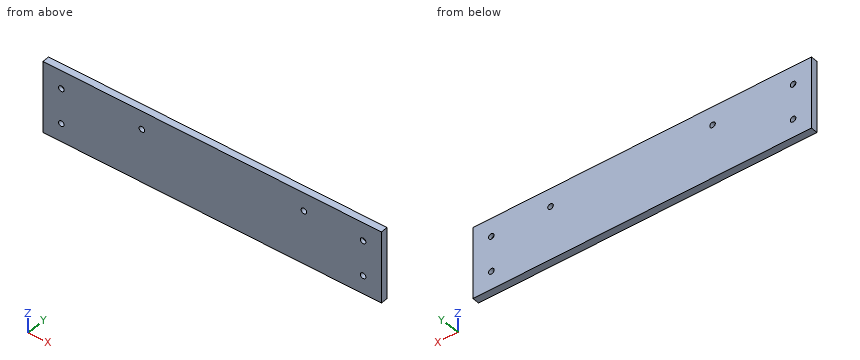
```python
from build123d import *

# Parameters (mm, degrees)
SKETCH1_W               = 305
SKETCH1_H               = 65
BOSS_EXTRUDE1_DEPTH     = 3.175
SKETCH4_R               = 2.5
CUT_EXTRUDE2_DEPTH      = 159.40243251
CUT_EXTRUDE3_DEPTH      = 157.053908955
CUT_EXTRUDE3_DEPTH_BACK = 157.053908955
SKETCH5_R               = 2.5


with BuildPart() as part:
    # Sketch1 → Boss-Extrude1 (new, symmetric)
    with BuildSketch(Plane(origin=(0, 0, 0), x_dir=(1, 0, 0), z_dir=(0, 1, 0))):
        Rectangle(SKETCH1_W, SKETCH1_H)
    extrude(amount=BOSS_EXTRUDE1_DEPTH, both=True)

    # Sketch4 → Cut-Extrude2 (cut, symmetric)
    with BuildSketch(Plane(origin=(-2.5, 0, 0), x_dir=(-1, 0, 0), z_dir=(0, -1, 0))):
        with Locations(Location((133.48, -15.98, 0), (0, 0, 90))):
            Circle(SKETCH4_R)
        with Locations(Location((133.48, 15.98, 0), (0, 0, 270))):
            Circle(SKETCH4_R)
    cut_extrude2 = extrude(amount=CUT_EXTRUDE2_DEPTH, both=True, mode=Mode.SUBTRACT)

    # Mirror2: Cut-Extrude2 across plane
    add(cut_extrude2.mirror(Plane(origin=(0, 0, 0), x_dir=(0, 0, 1), z_dir=(1, 0, 0))), mode=Mode.SUBTRACT)

    # Sketch5 → Cut-Extrude3 (cut, two sides: drawn at the far end of the back side and taken through both)
    with BuildSketch(Plane(origin=(0, 3.175, 0), x_dir=(1, 0, 0), z_dir=(0, 1, 0)).offset(-CUT_EXTRUDE3_DEPTH_BACK)):
        with Locations(Location((82.64, -15.98, 0), (0, 0, 270))):
            Circle(SKETCH5_R)
        with Locations(Location((-63.41, -15.98, 0), (0, 0, 270))):
            Circle(SKETCH5_R)
    extrude(amount=CUT_EXTRUDE3_DEPTH + CUT_EXTRUDE3_DEPTH_BACK, mode=Mode.SUBTRACT)


solid = part.part
```
Can you work these out from the model? Positions are in its coordinate system, mm. Coordinates: 2 decimals unless noted, no trailing zeros. Order: outer loops, then holes, each group sorted by start corner. A loop starts at its lowest first (then second) coordinate and runs counter-clockwise, first axis right, second up. Notation, with made-up numbers: (71.5, 31.25) - (120.5, 31.25) arc R29 cw to (120.5, 68.25) - close; hole circle Ø9 at (-31, -37). An arc over 180 degrees is marked (long way). Answer in a Markdown table with one row per item.
1. For pin 1 (4 mm diameter, centred on x = 135.98, z = -15.98, fed in from -Y), with a flat end and sliding along its axis, tell me the tip position at first contact or that it passes through.
Reply:
| item | result |
|---|---|
| pin 1 | passes through |
2. Suppose I cut it at C-C (x = 82.64). Please give me the cut outline in (y, z) (3 decimals), and give its area (3 significant figures).
Reply:
| item | result |
|---|---|
| outline | (-3.175, -32.5) - (3.175, -32.5) - (3.175, 13.48) - (-3.175, 13.48) - close; (-3.175, 18.48) - (3.175, 18.48) - (3.175, 32.5) - (-3.175, 32.5) - close |
| area | 381 mm^2 |
3. Suppose I cut it at A-A (z = -15.98). Please give me the cut outline in (x, y) (3 decimals), and give its area (3 significant figures).
Reply:
| item | result |
|---|---|
| outline | (-152.5, -3.175) - (-138.48, -3.175) - (-138.48, 3.175) - (-152.5, 3.175) - close; (-133.48, -3.175) - (133.48, -3.175) - (133.48, 3.175) - (-133.48, 3.175) - close; (138.48, -3.175) - (152.5, -3.175) - (152.5, 3.175) - (138.48, 3.175) - close |
| area | 1,870 mm^2 |
4. If I drill on line 1 along X through (y, z) = (1.7, 15.98); line 2 along X through (y, z) = (0, -15.98); line 3 along Z through (x, y) = (-135.98, 1.3), over which ranges is the centre line in solid material (lowest first)?
Reply:
| item | result |
|---|---|
| line 1 | x = -152.5 to -138.48, -133.48 to -65.91, -60.91 to 80.14, 85.14 to 133.48, 138.48 to 152.5 |
| line 2 | x = -152.5 to -138.48, -133.48 to 133.48, 138.48 to 152.5 |
| line 3 | z = -32.5 to -18.48, -13.48 to 13.48, 18.48 to 32.5 |
5. Suppose I cut it at B-B (x = 135.98). Please give me the cut outline in (y, z) (3 decimals), and give its area (3 significant figures).
Reply:
| item | result |
|---|---|
| outline | (-3.175, -32.5) - (3.175, -32.5) - (3.175, -18.48) - (-3.175, -18.48) - close; (-3.175, -13.48) - (3.175, -13.48) - (3.175, 13.48) - (-3.175, 13.48) - close; (-3.175, 18.48) - (3.175, 18.48) - (3.175, 32.5) - (-3.175, 32.5) - close |
| area | 349 mm^2 |
